from build123d import *

# Parameters (mm, degrees)
F0_R           = 7
F1_DEPTH       = 12
F2_D           = 5.5
F2_CBORE_D     = 9
F2_CBORE_DEPTH = 3
F4_DEPTH       = 8


with BuildPart() as f1:
    # F0 (on Right) → F1 (new body)
    with BuildSketch(Plane.YZ):
        Circle(F0_R)
    extrude(amount=F1_DEPTH)

    # F2 (through all)
    with Locations(Plane(origin=(0, 0, 0), x_dir=(0, 1, 0), z_dir=(-1, 0, 0))):
        with Locations((0, 0)):
            CounterBoreHole(F2_D / 2, F2_CBORE_D / 2, F2_CBORE_DEPTH)

    # F3 (on face) → F4 (cut)
    with BuildSketch(Plane.YZ.offset(12)):
        with BuildLine():
            ThreePointArc((5.467969, 4.370506), (0, 7), (-5.467969, 4.370506))
            ThreePointArc((-5.467969, 4.370506), (0, 3.3), (5.467969, 4.370506))
        make_face()
    extrude(amount=-F4_DEPTH, mode=Mode.SUBTRACT)


solid = f1.part
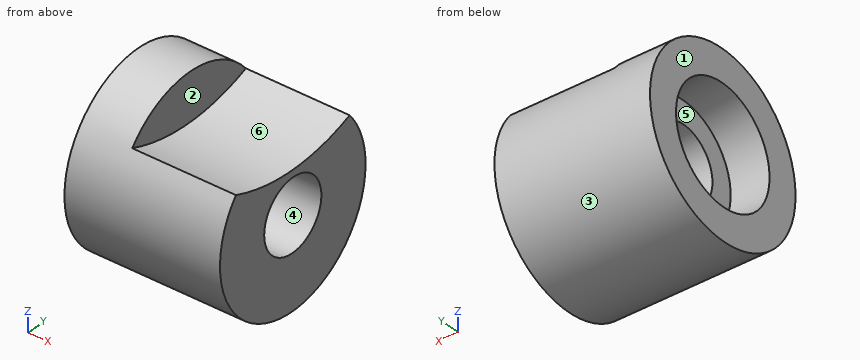
Part model, mm, in its own coordinate system. Face numbers are marked on the shaded views. A direction names the side the tool comes from. Coordinates: 2 decimals unless noted, no trailing zeros. Write each loop counter-clockwise with the first axis right and the second up, starting at its lowest first coordinate (ties: lowest second). Pieces come first, ordered by that corner, then holes. Notation, with made-up numbers: (-23, 0.25) - (1, 0.25) arc R31 ccw to (1, 32.25) - close; hole circle Ø1 at (33.25, 47). An arc over 180 degrees is marked (long way). Put each result on its own line as item: value.
1. Band-saw the part on A-A (z = 0). Write the cut outline in (x, y), then the cut area to 3 significant figures.
Final values:
outline: (0, -7) - (12, -7) - (12, -2.75) - (3, -2.75) - (3, -4.5) - (0, -4.5) - close; (0, 4.5) - (3, 4.5) - (3, 2.75) - (12, 2.75) - (12, 7) - (0, 7) - close
area: 91.5 mm²
2. 3-axis set-ups, long thin cutter, end or side, ignore diameter. For the marked faces 4, 5 and 6: which of +Z, -Z, +X, -X, +Y, -Y reach the whole face in a straight line?
Final values:
face 4: +X, -X
face 5: -X
face 6: +Z, +X
3. Band-saw the part on B-B (y = 0). Write the cut outline in (x, z), then the cut area to 3 significant figures.
Final values:
outline: (0, -7) - (12, -7) - (12, -2.75) - (3, -2.75) - (3, -4.5) - (0, -4.5) - close; (0, 4.5) - (3, 4.5) - (3, 2.75) - (12, 2.75) - (12, 3.3) - (4, 3.3) - (4, 7) - (0, 7) - close
area: 61.9 mm²
4. Two-plate mould, pull along Y, no slides. Class the marked faces 1, 2 and 3: +Y half, -Y half, draft (parallel to the pull), parting line (faces both ways), or undercut.
Final values:
face 1: draft
face 2: undercut
face 3: parting line
5. Flat gauge pins, fed straight in: pin 1 Ø6 at (x, y) = (4.5, -4) entering from -Z; pin 2 Ø1.1 at (y, z) = (1.5, 6) entering from +X; pin 3 Ø5 at (x, z) = (5.5, 3) entering from +Y. Where does each tip first touch, or does it go through?
Final values:
pin 1: stops at z = -6.93
pin 2: stops at x = 4
pin 3: stops at y = 6.98
6. Band-saw the part on D-D (z = -1.75). Write the cut outline in (x, y), then the cut area to 3 significant figures.
Final values:
outline: (0, -6.78) - (12, -6.78) - (12, -2.12) - (3, -2.12) - (3, -4.15) - (0, -4.15) - close; (0, 4.15) - (3, 4.15) - (3, 2.12) - (12, 2.12) - (12, 6.78) - (0, 6.78) - close
area: 99.6 mm²
7. Band-saw the part on C-C (x = 2.75). Write the cut outline in (y, z), then the cut area to 3 significant figures.
Final values:
outline: circle Ø14 at (0, 0); hole circle Ø9 at (0, 0)
area: 90.3 mm²
8. Probe line 1 along Z through (x, y) = (1.2, 0); line 2 along X through (y, z) = (2.25, -3.5); line 3 along Z through (x, y) = (11.5, 2). List the from-to ranges inside material, lowest first. Write a range as [from, to].
Final values:
line 1: z = [-7, -4.5], [4.5, 7]
line 2: x = [3, 12]
line 3: z = [-6.71, -1.89], [1.89, 3.44]
